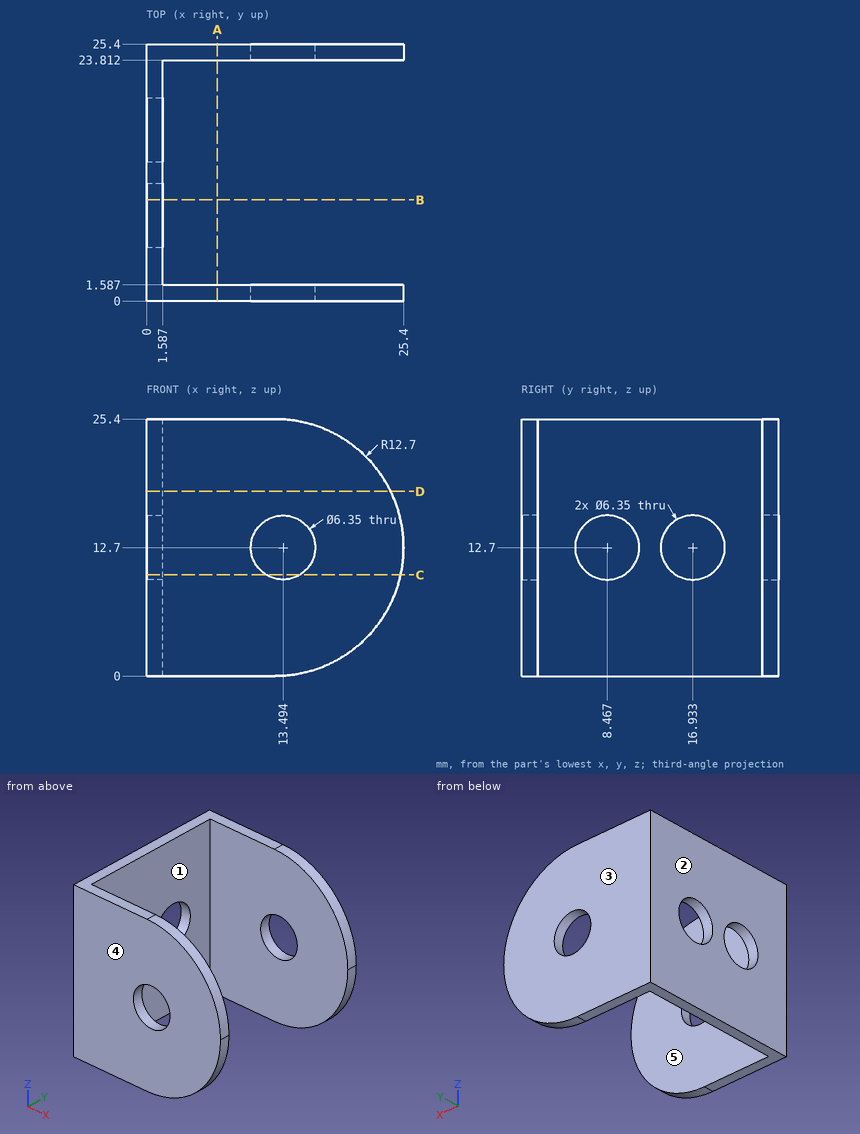
Geometry: see drawing. Coordinates: mm, zero at the bounding-box minimum. A direction names the side the tool comes from. Give positions to 0.01 mm unless a question says otherwise; leave off trailing zeros. Order: outer loops, then holes, each group sorted by start corner. A loop starts at its lowest first (then second) coordinate and runs counter-clockwise, first axis right, second up. Notation, with made-up numbers: (-33, -30) - (24, -30) arc R6 cw to (24, -23) - close; hole circle Ø4 at (68, -17.5). An arc over 180 degrees is marked (long way). One line per item, written item: value.
1. Draft query along Y for the marked faces 3, 4 and 5. Return one class per face: released by +Y, released by -Y, zero draft, split by the parting line, or undercut.
Determined:
face 3: released by +Y
face 4: released by -Y
face 5: undercut
2. Cut plane D-D, the plane z = 18.25. Output: boundary loops of the cut face in (x, y), and give its area (3 significant figures).
Determined:
outline: (0, 0) - (24.12, 0) - (24.12, 1.59) - (1.59, 1.59) - (1.59, 23.81) - (24.12, 23.81) - (24.12, 25.4) - (0, 25.4) - close
area: 112 mm2
3. Line query: probe 1 along Y at (x, z) = (0.65, 12.7); probe 2 along Y at (x, z) = (12.75, 20); probe 3 along X at (y, z) = (0.7, 12.7). Output: solid intervals per line, ascending.
Determined:
probe 1: 0 to 5.29, 11.64 to 13.76, 20.11 to 25.4
probe 2: 0 to 1.59, 23.81 to 25.4
probe 3: 0 to 10.32, 16.67 to 25.4
4. Cut plane A-A, the plane x = 7. Output: boundary loops of the cut face in (y, z).
Determined:
outline: (0, 0) - (1.59, 0) - (1.59, 25.4) - (0, 25.4) - close; (23.81, 0) - (25.4, 0) - (25.4, 25.4) - (23.81, 25.4) - close
5. Cut plane C-C, the plane z = 10. Output: boundary loops of the cut face in (x, y) (1 decimal).
Determined:
outline: (0, 0) - (11.8, 0) - (11.8, 1.6) - (1.6, 1.6) - (1.6, 6.8) - (0, 6.8) - close; (0, 10.1) - (1.6, 10.1) - (1.6, 15.3) - (0, 15.3) - close; (0, 18.6) - (1.6, 18.6) - (1.6, 23.8) - (11.8, 23.8) - (11.8, 25.4) - (0, 25.4) - close; (15.2, 0) - (25.1, 0) - (25.1, 1.6) - (15.2, 1.6) - close; (15.2, 23.8) - (25.1, 23.8) - (25.1, 25.4) - (15.2, 25.4) - close
6. Cut plane B-B, the plane y = 10. Output: boundary loops of the cut face in (x, z).
Determined:
outline: (0, 0) - (1.59, 0) - (1.59, 9.92) - (0, 9.92) - close; (0, 15.48) - (1.59, 15.48) - (1.59, 25.4) - (0, 25.4) - close
7. Reachability of the marked faces 1 and 2 from +Z, -Z, +X, -X, +Y, -Y: full face, straight path, thin tool, end or side. Return the list, or none.
Determined:
face 1: +Z, -Z, +X
face 2: +Z, -Z, -X, +Y, -Y
8. Pin query (flat end, axial travel): pin 1 Ø5.5 at (x, z) = (13.49, 12.7) entering from +Y; pin 2 Ø11 at (y, z) = (9.5, 10) entering from +X. Return the tip coordinate at first contact, or that it passes through.
Determined:
pin 1: through
pin 2: x = 1.59
